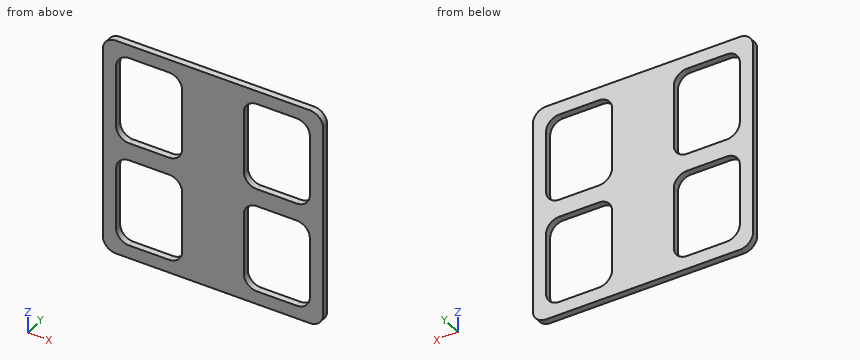
from build123d import *

# Parameters (mm, degrees)
EXTRUDE_1_DEPTH = 15


with BuildPart() as part:
    # 草图1 → 凸台-拉伸1 (new body)
    with BuildSketch(Plane(origin=(0, 0, 0), x_dir=(1, 0, 0), z_dir=(0, 1, 0))):
        with BuildLine():
            Line((220, 250), (-220, 250))
            ThreePointArc((-220, 250), (-241.213203436, 241.213203436), (-250, 220))
            Line((-250, 220), (-250, -220))
            ThreePointArc((-250, -220), (-241.213203436, -241.213203436), (-220, -250))
            Line((-220, -250), (220, -250))
            ThreePointArc((220, -250), (241.213203436, -241.213203436), (250, -220))
            Line((250, -220), (250, 220))
            ThreePointArc((250, 220), (241.213203436, 241.213203436), (220, 250))
        make_face()
        with BuildLine():
            Line((-100, 20), (-190, 20))
            ThreePointArc((-190, 20), (-211.213203436, 28.786796564), (-220, 50))
            Line((-220, 50), (-220, 190))
            ThreePointArc((-220, 190), (-211.213203436, 211.213203436), (-190, 220))
            Line((-190, 220), (-100, 220))
            ThreePointArc((-100, 220), (-78.786796564, 211.213203436), (-70, 190))
            Line((-70, 190), (-70, 50))
            ThreePointArc((-70, 50), (-78.786796564, 28.786796564), (-100, 20))
        make_face(mode=Mode.SUBTRACT)
        with BuildLine():
            Line((220, 50), (220, 190))
            ThreePointArc((220, 190), (211.213203436, 211.213203436), (190, 220))
            Line((190, 220), (100, 220))
            ThreePointArc((100, 220), (78.786796564, 211.213203436), (70, 190))
            Line((70, 190), (70, 50))
            ThreePointArc((70, 50), (78.786796564, 28.786796564), (100, 20))
            Line((100, 20), (190, 20))
            ThreePointArc((190, 20), (211.213203436, 28.786796564), (220, 50))
        make_face(mode=Mode.SUBTRACT)
        with BuildLine():
            Line((-220, -50), (-220, -190))
            ThreePointArc((-220, -190), (-211.213203436, -211.213203436), (-190, -220))
            Line((-190, -220), (-100, -220))
            ThreePointArc((-100, -220), (-78.786796564, -211.213203436), (-70, -190))
            Line((-70, -190), (-70, -50))
            ThreePointArc((-70, -50), (-78.786796564, -28.786796564), (-100, -20))
            Line((-100, -20), (-190, -20))
            ThreePointArc((-190, -20), (-211.213203436, -28.786796564), (-220, -50))
        make_face(mode=Mode.SUBTRACT)
        with BuildLine():
            Line((100, -20), (190, -20))
            ThreePointArc((190, -20), (211.213203436, -28.786796564), (220, -50))
            Line((220, -50), (220, -190))
            ThreePointArc((220, -190), (211.213203436, -211.213203436), (190, -220))
            Line((190, -220), (100, -220))
            ThreePointArc((100, -220), (78.786796564, -211.213203436), (70, -190))
            Line((70, -190), (70, -50))
            ThreePointArc((70, -50), (78.786796564, -28.786796564), (100, -20))
        make_face(mode=Mode.SUBTRACT)
    extrude(amount=EXTRUDE_1_DEPTH)


solid = part.part
Part model, mm, in its own coordinate system. Coordinates: 2 decimals unless noted, no trailing zeros. Loops run counter-clockwise (first coordinate to the right, second up) from the corner with the lowest first, then second, coordinate; pieces in that order, holes last. Notation, with made-up numbers: M 87,48.5 L 142,48.5 A22 ccw 142,61.5 Z; hole C -12,73 d7. An arc over 180 degrees is marked long. Use a Markdown table: item, result. Add a question column.
Q1. Probe L1, parallel to X at y = 9, z = 90; L2, parallel to Z at x = -117, y = 7.5; L3, parallel to Z at x = -200.5, y = 4.5. List the from-to ranges inside material, lowest first.
Q2. Cut at C-C (y = 10.5). Give the number of separate pieces and of enclosed holes in the cut face, and give its area (3 significant figures).
Q3. Cut at B-B (x = 207). Write the cut outline in (y, z).
Q4. Cut at A-A (z = 85). Write the cut outline in (x, y), and give its area (3 significant figures).
Worked out:
| question | item | result |
|---|---|---|
| 1 | L1 | x = -250 to -220, -70 to 70, 220 to 250 |
| 1 | L2 | z = -250 to -220, -20 to 20, 220 to 250 |
| 1 | L3 | z = -250 to -218.1, -21.9 to 21.9, 218.1 to 250 |
| 2 | separate pieces | 1 |
| 2 | enclosed holes | 4 |
| 2 | area | 132,000 mm2 |
| 3 | outline | M 0,-250 L 15,-250 L 15,-214.72 L 0,-214.72 Z; M 0,-25.28 L 15,-25.28 L 15,25.28 L 0,25.28 Z; M 0,214.72 L 15,214.72 L 15,250 L 0,250 Z |
| 4 | outline | M -250,0 L -220,0 L -220,15 L -250,15 Z; M -70,0 L 70,0 L 70,15 L -70,15 Z; M 220,0 L 250,0 L 250,15 L 220,15 Z |
| 4 | area | 3,000 mm2 |
